Input: part model. Units: mm. Frame: model coordinates. A direction names the side the tool comes from. Round coordinates to 2 decimals unless told otherwise and drop trailing zeros. Order: outer loops, then holes, each group sorted by start corner. A loop starts at its lowest first (then second) coordinate and runs counter-clockwise, first axis right, second up. Notation, with made-up numbers: (82.5, -3.75) -> (114.5, -3.75) arc R8 ccw to (114.5, 10.25) -> close; hole circle Ø4 at (-7, 80). An arc over 180 degrees is marked (long way). Use a Markdown table: item, result.
Autodesk Inventor part; units mm, degrees
ref_plane "РабПлоскость1" through (0, 0, 3.05) normal (0, 0, 1) x (1, 0, 0)
ref_plane "YZ Plane" through (0, 0, 0) normal (1, 0, 0) x (0, 1, 0)
ref_plane "XZ Plane" through (0, 0, 0) normal (0, 1, 0) x (-1, 0, 0)
sketch "Эскиз2" plane through (0, 0, 0) normal (0, 0, 1) x (1, 0, 0)
  line L0 (0, 0) -> (10.05, 0)
  line L1 (10.05, 0) -> (10.05, 3.4)
  line L2 (10.05, 3.4) -> (0, 3.4)
  line L3 (0, 3.4) -> (0, 0)
  line L4 (10.05, 0) -> (31.15, 0)
  line L5 (31.15, 0) -> (31.15, 18.1)
  line L6 (31.15, 18.1) -> (10.05, 18.1)
  line L7 (10.05, 18.1) -> (10.05, 0)
  line L8 (31.15, 0) -> (41.2, 0)
  line L9 (41.2, 0) -> (41.2, 3.4)
  line L10 (41.2, 3.4) -> (31.15, 3.4)
  line L11 (31.15, 3.4) -> (31.15, 0)
  line L12 (20.6, 18.1) -> (20.6, 7.55)
  circle A0 centre (20.6, 7.55) radius 8.55
  line L13 (7, 0) -> (26, 0)
  line L14 (12.05, 7.55) -> (29.15, 7.55)
  line L15 (29.15, 7.55) -> (29.15, 0)
  line L16 (29.15, 0) -> (12.05, 0)
  line L17 (12.05, 0) -> (12.05, 7.55)
  point P0 (31.15, 3.4)
  point P1 (16.5875, 0)
  point P2 (24.6125, 0)
  point P3 (12.05, 0)
  point P4 (12.05, 7.55)
  point P5 (29.15, 0)
  dimension "d14" = 17.1
  dimension "d0" = 10.05
  dimension "d1" = 21.1
  dimension "d2" = 18.1
  dimension "d3" = 3.4
  dimension "d4" = 10.05
  dimension "d13" = 10.55
  dimension "d15" = 3.4
extrude "Выдавливание1" add sketch "Эскиз2" along normal blind 6.1 contours L3 L2 L1 L0 | L1 L7 L6 L12 A0 L17 L4 | L6 L5 L4 L15 A0 L12 | L10 L9 L8 L5
sketch "Эскиз4" plane through (0, 0, 6.1) normal (0, 0, 1) x (1, 0, 0)
  line L0 (0, 0) -> (12.05, 0)
  line L1 (12.05, 0) -> (12.05, 7.55)
  arc A0 (29.15, 7.55) -> (12.05, 7.55) centre (20.6, 7.55) ccw
  line L2 (29.15, 7.55) -> (29.15, 0)
  line L3 (41.2, 0) -> (41.2, 3.4)
  line L4 (41.2, 3.4) -> (31.15, 3.4)
  line L5 (31.15, 3.4) -> (31.15, 18.1)
  line L6 (31.15, 18.1) -> (10.05, 18.1)
  line L7 (10.05, 18.1) -> (10.05, 3.4)
  line L8 (10.05, 3.4) -> (0, 3.4)
  line L9 (0, 3.4) -> (0, 0)
  line L10 (12.05, 0) -> (29.15, 0)
  line L11 (29.15, 0) -> (41.2, 0)
extrude "Выдавливание3" add sketch "Эскиз4" along normal blind 2
ref_plane "РабПлоскость1" through (0, 0, 3.05) normal (0, 0, 1) x (1, 0, 0)
mirror "Зеркальное отражение2" about plane through (0, 0, 3.05) normal (0, 0, 1) of "Выдавливание3"
fillet "Сопряжение2" radius 10.55 2 edges at (31.15, 18.1, 3.05) (10.05, 18.1, 3.05)
sketch "Эскиз6" plane through (31.15, 3.4, 8.1) normal (0, 1, 0) x (1, 0, 0)
  line L0 (10.05, 10.1) -> (10.05, 0)
  line L1 (10.05, 5.05) -> (0, 5.05)
  line L2 (0, 10.1) -> (0, 0)
  line L3 (-21.1, 10.1) -> (-21.1, 0)
  line L4 (-21.1, 5.05) -> (-31.15, 5.05)
  line L5 (-31.15, 0) -> (-31.15, 10.1)
  line L6 (-26.125, 5.05) -> (-26.1, 5.05)
  line L7 (5.025, 5.05) -> (5, 5.05)
  point P0 (-31.15, 8.1)
  dimension "d35" = 0.025
  dimension "d36" = 0.025
hole "Отверстие2" at (5.05, 3.4, 3.05) at (36.15, 3.4, 3.05) direction (0, -1, 0) diameter 3.2 end through all countersink diameter 6 countersink angle 90
sketch "Эскиз7" plane through (0, 0, 8.1) normal (0, -1, 0) x (1, 0, 0)
  line L0 (0, -10.1) -> (0, 0)
  line L1 (41.2, -10.1) -> (31.15, -10.1)
  line L2 (0, 0) -> (41.2, 0)
  line L3 (41.2, 0) -> (41.2, -10.1)
  line L4 (41.2, -10.1) -> (0, -10.1)
  line L5 (0, -10.1) -> (0, 0)
  line L6 (0, 0) -> (2, 0)
  line L7 (2, 0) -> (2, -2)
  line L8 (2, -2) -> (39.2, -2)
  line L9 (39.2, -2) -> (39.2, -8.1)
  line L10 (39.2, -8.1) -> (2, -8.1)
  line L11 (2, -8.1) -> (2, -2)
  line L12 (41.2, -10.1) -> (41.2, 0)
  line L13 (41.2, -10.1) -> (39.2, -10.1)
  line L14 (39.2, -10.1) -> (39.2, -8.1)
  point P0 (0, -8.1)
  dimension "d37" = 2
  dimension "d38" = 2
  dimension "d39" = 2
  dimension "d40" = 2
extrude "Выдавливание4" add sketch "Эскиз7" along normal blind 3.7 contours L0 L2 L7 L11 L10 L14 L1 L4 | L2 L3 L1 L14 L9 L8 L7
sketch "Эскиз8" plane through (0, 0, 8.1) normal (0, 0, 1) x (1, 0, 0)
  arc A0 (31.15, 7.55) -> (10.05, 7.55) centre (20.6, 7.55) ccw
  point P0 (0, 0)
hole "Отверстие3" at (20.6, 7.55, 8.1) direction (0, 0, -1) diameter 8 end through all
fillet "Сопряжение3" radius 5.05 2 edges at (0, -0.15, 8.1) (0, -0.15, -2)
fillet "Сопряжение4" radius 5.05 2 edges at (41.2, -0.15, 8.1) (41.2, -0.15, -2)
fillet "Сопряжение5" radius 3.05 2 edges at (2, -1.85, 6.1) (2, -1.85, 0)
fillet "Сопряжение6" radius 3.05 2 edges at (39.2, -1.85, 0) (39.2, -1.85, 6.1)
equation "\"d0\" = d4"
equation "\"d15\" = d3"
equation "\"Радиус_гибки\" = Толщина"
equation "\"Ширина_просечки\" = Толщина"
equation "\"Глубина_просечки\" = 0.5 * Толщина"
equation "\"Размер_просечки\" = 4 * Толщина"
equation "\"Мин_остаток\" = 2 * Толщина"
equation "\"Радиус_перехода\" = Радиус_гибки"
equation "\"Радиус_Якоби\" = Толщина"
equation "\"Размер_зазора\" = Толщина"
properties part number "Крышка стойки подшипника"
1) Draft query along X for faces 3 (the face through (8.4, 3.4, 3)), 4 (the face through (13.06, 14.93, 2.98)), 5 (the face through (20.412, 16.098, 3.007)). Return one class per face: released by +X, released by -X, zero draft, split by the parting line, or undercut.
Answer key:
| item | result |
|---|---|
| face 3 | zero draft |
| face 4 | released by -X |
| face 5 | undercut |
2) Contact query for flat-ended pins moving along their axis: P1, Ø5, axis at x = 38.5, z = 2.5, coming from the +Y side; P2, Ø1.8, axis at x = 5.5, z = 4, coming from the -Y side; P3, Ø3, axis at y = -1, z = 5.5, coming from the +X side. Output: stop coordinate, or through.
Answer key:
| item | result |
|---|---|
| P1 | stops at y = 3.4 |
| P2 | stops at y = 0 |
| P3 | stops at x = 41.11 |
3) Cut plane D-D on y = 9.25. Return loops of the section in (x, z).
Answer key:
| item | result |
|---|---|
| outline | (10.19, -2) -> (16.98, -2) -> (16.98, 0) -> (12.22, 0) -> (12.22, 6.1) -> (16.98, 6.1) -> (16.98, 8.1) -> (10.19, 8.1) -> close; (24.22, -2) -> (31.01, -2) -> (31.01, 8.1) -> (24.22, 8.1) -> (24.22, 6.1) -> (28.98, 6.1) -> (28.98, 0) -> (24.22, 0) -> close |
4) Ray query, probe 1 along X at (y, z) = (1.15, 3.05); probe 2 along X at (y, z) = (7.55, -1.25); probe 3 along Z at (x, y) = (14, 0.75). Return the intervals inside material, ascending.
Answer key:
| item | result |
|---|---|
| probe 1 | x = 0 to 3.45, 6.65 to 12.05, 29.15 to 34.55, 37.75 to 41.2 |
| probe 2 | x = 10.05 to 16.6, 24.6 to 31.15 |
| probe 3 | z = -2 to 0, 6.1 to 8.1 |
5) Cut plane B-B on x = 17.5. Return loops of the section in (y, z), and give its area (3 significant figures).
Answer key:
| item | result |
|---|---|
| outline | (-3.7, -2) -> (5.02, -2) -> (5.02, 0) -> (-3.7, 0) -> close; (-3.7, 6.1) -> (5.02, 6.1) -> (5.02, 8.1) -> (-3.7, 8.1) -> close; (10.08, -2) -> (17.63, -2) -> (17.63, 8.1) -> (10.08, 8.1) -> (10.08, 6.1) -> (15.52, 6.1) -> (15.52, 0) -> (10.08, 0) -> close |
| area | 78.0 mm^2 |
6) Cut plane A-A on y = 6. Return loops of the section in (x, z).
Answer key:
| item | result |
|---|---|
| outline | (10.05, -2) -> (16.91, -2) -> (16.91, 0) -> (12.05, 0) -> (12.05, 6.1) -> (16.91, 6.1) -> (16.91, 8.1) -> (10.05, 8.1) -> close; (24.29, -2) -> (31.15, -2) -> (31.15, 8.1) -> (24.29, 8.1) -> (24.29, 6.1) -> (29.15, 6.1) -> (29.15, 0) -> (24.29, 0) -> close |
7) Set-up query: faces 1 (the face through (28.14, 14.93, 3.12)), 2 (the face through (8, 0, 3)). Return all of +Z, -Z, +X, -X, +Y, -Y with unobstructed straight access to the full face (end or side cutting, diameter ignored); none if empty.
Answer key:
| item | result |
|---|---|
| face 1 | +Z, -Z, +X, +Y |
| face 2 | -Y |
